CAD build for the part. Positions are in the model's coordinates, mm. A direction names the side the tool comes from. Coordinates: 2 decimals unless noted, no trailing zeros. Loops run counter-clockwise (first coordinate to the right, second up) from the corner with the lowest first, then second, coordinate; pieces in that order, holes last. Notation, with made-up numbers: (76, 57.25) -> (101, 57.25) arc R19 ccw to (101, 75.25) -> close; hole circle Ø3 at (56, -30.5). An arc over 180 degrees is marked (long way). Answer as CSV lines item,"result". Start each with the question number.
```python
from build123d import *

# Parameters (mm, degrees)
F1_DEPTH    = 38
F3_DEPTH    = 50
F4_T4_DEPTH = 9
F4_T9_DEPTH = 9
F5_W        = 38
F5_H        = 14.5097850376
F6_DEPTH    = 25
F7_R        = 2
F8_R        = 1.5


# Not quite as in the source:
# - a fillet or chamfer that OpenCascade refuses, or shapes differently, is made with other operations: its cross-section is extruded or revolved along the edge and cut away or added


with BuildPart() as f1:
    # F0 (on Front) → F1 (new body)
    with BuildSketch(Plane.XZ):
        Polygon((0, 16.9122221599), (0, -11.0877778401), (1.5, -11.0877778401), (1.5, 14.4122221599), (3.5, 14.4122221599), (3.5, 3.4220071975), (5, 3.4220071975), (5, 6.7475574595), (5, 8.2475574595), (5, 16.9122221599), align=None)
        Polygon((11.4920105912, 8.2475574595), (5, 8.2475574595), (5, 6.7475574595), (11.9522421048, 6.7475574595), (15, 9.3381504056), (14.0667535676, 10.4360879209), align=None)
    extrude(amount=F1_DEPTH)

    # F2 (on face) → F3 (cut)
    with BuildSketch(Plane.XY.offset(16.9122221599)):
        Polygon((16.5792163461, -29), (16.5792163461, -19), (16.5792163461, -9), (5, -9), (5, -29), align=None)
    extrude(amount=-F3_DEPTH, mode=Mode.SUBTRACT)

    # F4: chamfer of 4 on 2 edges, made by hand


with BuildPart() as f4_tool2:
    # F4_s3 → F4_t4 (new body)
    with BuildSketch(Plane.XZ.offset(29)):
        Polygon((9, 6.7475574595), (5, 2.7475574595), (5, 6.7475574595), align=None)
    extrude(amount=F4_T4_DEPTH)

    split(bisect_by=Plane.XY.offset(3.4220071975), keep=Keep.TOP)


with BuildPart() as f1_1:
    add(f1.part)

    # F4_t1: union F4_tool2
    add(f4_tool2.part)


with BuildPart() as f4_tool7:
    # F4_s8 → F4_t9 (new body)
    with BuildSketch(Plane.XZ):
        Polygon((5, 2.7475574595), (9, 6.7475574595), (5, 6.7475574595), align=None)
    extrude(amount=F4_T9_DEPTH)

    split(bisect_by=Plane.XY.offset(3.4220071975), keep=Keep.TOP)


with BuildPart() as f1_2:
    add(f1_1.part)

    # F4_t6: union F4_tool7
    add(f4_tool7.part)

    # F5 (on face) → F6 (cut)
    with BuildSketch(Plane.YZ.offset(1.5)):
        with Locations((-19, -3.8328853213)):
            Rectangle(F5_W, F5_H)
    extrude(amount=-F6_DEPTH, mode=Mode.SUBTRACT)

    # F7
    f7_edges = [f1_2.edges().sort_by_distance(p)[0] for p in [
        (5, -33.5, 8.247557),
        (5, -4.5, 8.247557),
    ]]
    fillet(f7_edges, radius=F7_R)

    # F8
    f8_edges = [f1_2.edges().sort_by_distance(p)[0] for p in [
        (5, -19, 16.912222),
        (0, -19, 16.912222),
    ]]
    fillet(f8_edges, radius=F8_R)


solid = f1_2.part
```
Q1. Probe probe 1 along X at (y, z) = (-32, 8.5); probe 2 along X at (y, z) = (-18, 14); probe 3 along Z at (x, y) = (10.5, -30). List the from-to ranges inside material, lowest first. Write a range as from..to.
Q2. Which spindle directions (+Z, -Z, +X, -X, +Y, -Y) get a long thin tool onto all of the face, cutting with end or side? Do faces 1 (the flat face through (2, -19, 14.412)), 2 (the flat face through (9, -29, 7)), 3 (the flat face through (12.8, -4.44, 9.36)), 4 (the flat face through (10, -33, 6.748)). Say none if no direction does.
Q3. Saw through at A-A (x = 9.75). List the corners of the cut face in (y, z).
Q4. Pin check, flat tips, straight feed: pin 1 Ø5 at (x, y) = (10.5, -6.5) entering from +Z; pin 2 Ø1.5 at (x, y) = (11, -32.5) entering from -Z; pin 3 Ø3 at (y, z) = (-18, 7) entering from +X. Stop position of each tip, or through.
Q5. Saw through at D-D (z = 15). List the corners of the cut face in (x, y).
Q6. Saw through at B-B (z = 12.75). List the corners of the cut face in (x, y).
Q7. Saw through at C-C (y = -7). List the corners of the cut face in (x, z), and give its area (3 significant figures).
Ans:
1,probe 1,"x = 0..1.5, 3.5..6.03, 11.79..14.01"
1,probe 2,"x = 0..1.5, 3.5..5"
1,probe 3,"z = 6.75..8.25"
2,face 1,"-Z, +Y, -Y"
2,face 2,"+Z, -Z, +X"
2,face 3,"+Z, +Y, -Y"
2,face 4,"-Z, +X, +Y, -Y"
3,outline,"(-38, 6.75) -> (-29, 6.75) -> (-29, 8.25) -> (-38, 8.25) -> close; (-9, 6.75) -> (0, 6.75) -> (0, 8.25) -> (-9, 8.25) -> close"
4,pin 1,"stops at z = 9.53"
4,pin 2,"stops at z = 6.75"
4,pin 3,"stops at x = 5"
5,outline,"(0, -38) -> (5, -38) -> (5, 0) -> (0, 0) -> close"
6,outline,"(0, -38) -> (1.5, -38) -> (1.5, 0) -> (0, 0) -> close; (3.5, -38) -> (5, -38) -> (5, 0) -> (3.5, 0) -> close"
7,outline,"(0, 3.42) -> (1.5, 3.42) -> (1.5, 14.41) -> (3.5, 14.41) -> (3.5, 3.42) -> (5.67, 3.42) -> (9, 6.75) -> (11.95, 6.75) -> (15, 9.34) -> (14.07, 10.44) -> (11.49, 8.25) -> (7, 8.25) arc R2 cw to (5, 10.25) -> (5, 15.41) arc R1.5 ccw to (3.5, 16.91) -> (1.5, 16.91) arc R1.5 ccw to (0, 15.41) -> close"
7,area,"68.5 mm²"
